For this review, take the finished solid that the model builds, in its own axes (mm). A direction names the side the tool comes from. Round coordinates to 2 decimals unless told otherwise and drop trailing zeros. Write each loop counter-clockwise with the first axis right and the second up, starting at its lowest first coordinate (ties: lowest second). Pieces come first, ordered by that corner, then holes. Notation, with made-up numbers: (63, 77) -> (82, 77) arc R29 ccw to (82, 108) -> close; hole circle Ø3 at (0.5, 39). An arc over 180 degrees is marked (long way). Answer as CSV lines item,"result". Start each with the question number.
Item 1: Machinability: for faces 4 (the flat face through (0, 0, 0)), 5 (the conical face through (4.33, 13.49, 0.96)), which of the approach directions +Z, -Z, +X, -X, +Y, -Y give a long, thin tool a straight path to every point of the face, cutting with its end or side? Answer none if there is none.
Item 2: Take a section at C-C on y = 7. Give the boundary of the cut face in (x, z), then the cut area to 3 significant figures.
Item 3: Mouldability with a two-part tool opening along Y and no side actions: class faces 1 (the flat face through (3, 3.175, -8)), 2 (the cylindrical face through (5.796, 1.223, 7.559)), 3 (the flat face through (3, 20.447, 2)) as +Y half, -Y half, draft (parallel to the pull), parting line (faces both ways), or undercut.
Item 4: For pin 1 Ø3 at (x, z) = (-7.5, -7.5) entering from +Y; pin 2 Ø3 at (x, y) = (-0.5, 16.5) entering from +Z; pin 3 Ø3 at (x, y) = (2, 8.5) entering from +Z, all flat-tipped, find the tip position at first contact; note any pin that passes through.
Item 5: Take a section at D-D on y = 11.75. Give the boundary of the cut face in (x, z), then the cut area to 3 significant figures.
Item 6: Wall thickness on probe 1 along Y at (x, z) = (-0.5, -6.5); probe 2 along Z at (x, y) = (-4.75, 8.25); probe 3 along Z at (x, y) = (1, 15): over which ranges is each line inside the solid? List them lowest first. Write a range as from..to.
```python
from build123d import *

# Parameters (mm, degrees)
FILLET1_R     = 1.524
CHAMFER1_SIZE = 0.762


with BuildPart() as part:
    # Sketch1 → Revolve1 (revolve)
    with BuildSketch(Plane.XY, mode=Mode.PRIVATE) as revolve1_sk:
        with BuildLine():
            Line((0, 0), (-9.525, 0))
            Line((-9.525, 0), (-9.525, 3.175))
            Line((-9.525, 3.175), (-8.001, 3.175))
            Line((-8.001, 3.175), (-8.001, 4.699))
            Line((-8.001, 4.699), (-6.477, 4.699))
            Line((-6.477, 4.699), (-3.175, 18.923))
            Line((-3.175, 18.923), (-4.131690787, 18.923))
            ThreePointArc((-4.131690787, 18.923), (-4.893690787, 19.685), (-4.131690787, 20.447))
            Line((-4.131690787, 20.447), (-3.369690787, 20.447))
            ThreePointArc((-3.369690787, 20.447), (-4.399409051, 25.63639864), (0, 28.575))
            Line((0, 28.575), (0, 0))
        make_face()
    revolve(revolve1_sk.sketch.rotate(Axis((0, 0, 0), (0, 1, 0)), 270), axis=Axis((0, 0, 0), (0, 1, 0)))

    # Fillet1
    fillet1_edges = [part.edges().sort_by_distance(p)[0] for p in [
        (0, 4.699, 8.001),
    ]]
    fillet(fillet1_edges, radius=FILLET1_R - 0.0001)  # a hair under: the kernel refuses the full size

    # Chamfer1
    chamfer1_edges = [part.edges().sort_by_distance(p)[0] for p in [
        (0, 3.175, 9.525),
    ]]
    chamfer(chamfer1_edges, length=CHAMFER1_SIZE)


solid = part.part
```
Output values:
1,face 4,"+Z, -Z, +X, -X, -Y"
1,face 5,"none"
2,outline,"circle Ø11.89 at (0, 0)"
2,area,"111 mm^2"
3,face 1,"+Y half"
3,face 2,"draft"
3,face 3,"undercut"
4,pin 1,"stops at y = 2.83"
4,pin 2,"stops at z = 4.07"
4,pin 3,"stops at z = 5.77"
5,outline,"circle Ø9.68 at (0, 0)"
5,area,"73.6 mm^2"
6,probe 1,"y = 0..4.7"
6,probe 2,"z = -3.06..3.06"
6,probe 3,"z = -3.96..3.96"
